Could you check a few things on this model? Use its own coordinates, in mm. A direction names the side the tool comes from. Give positions to 0.01 mm unless a question says otherwise; leave off trailing zeros. Order: outer loops, then holes, each group sorted by start corner. A loop starts at its lowest first (then second) coordinate and runs counter-clockwise, first axis right, second up. Notation, with made-up numbers: M 69,71 L 90,71 A14 cw 90,95 Z; hole C 7.5,7 d4. An arc over 180 degrees is marked long. Answer in a Markdown table with one row per item. Add a question column.
```python
from build123d import *

# Parameters (mm, degrees)
F1_DEPTH       = 101.6
F3_D           = 4.7752
F3_CBORE_D     = 9.525
F3_CBORE_DEPTH = 3.175
F5_D           = 4.7752
F5_CBORE_D     = 9.525
F5_CBORE_DEPTH = 3.175
F7_D           = 6.35
F8_SIZE        = 44.45
F9_R           = 12.7


with BuildPart() as f1:
    # F0 (on Front) → F1 (new body)
    with BuildSketch(Plane.XZ):
        Polygon((0, 9.525), (0, 0), (119.0752, 0), (119.0752, 10.549193), (68.2752, 10.549193), (68.2752, 55.613711), (61.9252, 55.613711), (61.9252, 10.139516), (57.15, 10.139516), (57.15, 55.40887), (50.8, 55.40887), (50.8, 9.525), align=None)
    extrude(amount=F1_DEPTH)

    # F3 (through all)
    with Locations(Plane.XY.offset(9.525)):
        with Locations((22.530584, -12.7), (24.763316, -88.9)):
            CounterBoreHole(F3_D / 2, F3_CBORE_D / 2, F3_CBORE_DEPTH)

    # F5 (through all)
    with Locations(Plane.XY.offset(10.549193)):
        with Locations((90.809768, -12.7), (93.242841, -88.9)):
            CounterBoreHole(F5_D / 2, F5_CBORE_D / 2, F5_CBORE_DEPTH)

    # F7 (through all)
    with Locations(Plane(origin=(50.8, 0, 0), x_dir=(0, -1, 0), z_dir=(-1, 0, 0))):
        with Locations((47.544591, 46.355)):
            Hole(F7_D / 2)

    # F8
    f8_edges = [f1.edges().sort_by_distance(p)[0] for p in [
        (53.975, 0, 55.40887),
        (53.975, -101.6, 55.40887),
        (65.1002, -101.6, 55.613711),
        (65.1002, 0, 55.613711),
    ]]
    chamfer(f8_edges, length=F8_SIZE)

    # F9
    f9_edges = [f1.edges().sort_by_distance(p)[0] for p in [
        (0, 0, 4.7625),
        (0, -101.6, 4.7625),
        (119.0752, -101.6, 5.274597),
        (119.0752, 0, 5.274597),
    ]]
    fillet(f9_edges, radius=F9_R)


solid = f1.part
```
1. Thinking about a two-plate mould opening in Y: for faces 1 (the flat face through (59, 0, 6)), 2 (the flat face through (59, -101.6, 6)), 3 (the flat face through (60, -50, 10.14)), 4 (the flat face through (95, -91, 7.374)), which applies, pulls with the +Y half, pulls with the -Y half, needs draft (parallel to the pull), parting line crosses it, or undercut?
2. Suppose I cut it at B-B on y = -68.5. List the corners of the cut face in (x, z) for me (3 decimals), plus the area to 3 significant figures.
3. Suppose I cut it at C-C on x = 48. List the corners of the cut face in (y, z) for me (3 decimals), plus the area to 3 significant figures.
4. Will these pins go through, and if not, where does the flat tip stop? P1, Ø1.5, axis at x = 51, z = 28, coming from the +Y side; P2, Ø7.5, axis at x = 23, y = -14, coming from the +Z side (3 decimals); P3, Ø5.5, axis at x = 22.53, y = -12.7, coming from the +Z side.
5. If I drill on line 1 along X through (y, z) = (-65.5, 38.5); line 2 along Y through (x, z) = (24, 4), over which ranges is the centre line in solid material (lowest first)? Write a range as [from, to].
6. Suppose I cut it at D-D on z = 14. List the corners of the cut face in (x, y) for me.
7. Suppose I cut it at A-A on z = 30. List the corners of the cut face in (x, y) for me.
8. For faces 5 (the flat face through (61.925, -50, 28)), 6 (the cylindrical face through (115.256, -3.622, 5.348)), 7 (the flat face through (26, -50, 9.525)), 8 (the flat face through (93, -15, 7.374)), 9 (the flat face through (68.275, -50, 28)), which set-ups out of +Z, -Z, +X, -X, +Y, -Y let a thin tool reach every point of the face, with its end or its side?
Findings below:
| question | item | result |
|---|---|---|
| 1 | face 1 | pulls with the +Y half |
| 1 | face 2 | pulls with the -Y half |
| 1 | face 3 | needs draft |
| 1 | face 4 | undercut |
| 2 | outline | M 0,0 L 119.075,0 L 119.075,10.549 L 68.275,10.549 L 68.275,44.264 L 61.925,44.264 L 61.925,10.14 L 57.15,10.14 L 57.15,44.059 L 50.8,44.059 L 50.8,9.525 L 0,9.525 Z |
| 2 | area | 1,630 mm2 |
| 3 | outline | M -101.6,0 L 0,0 L 0,9.525 L -101.6,9.525 Z |
| 3 | area | 968 mm2 |
| 4 | P1 | y = -16.29 |
| 4 | P2 | z = 9.525 |
| 4 | P3 | z = 6.35 |
| 5 | line 1 | [50.8, 57.15], [61.93, 68.28] |
| 5 | line 2 | [-101.6, -91.16], [-86.64, -14.58], [-10.82, 0] |
| 6 | outline | M 50.8,-98.56 L 57.15,-98.56 L 57.15,-3.04 L 50.8,-3.04 Z; M 61.93,-98.76 L 68.28,-98.76 L 68.28,-2.84 L 61.93,-2.84 Z |
| 7 | outline | M 50.8,-82.56 L 57.15,-82.56 L 57.15,-19.04 L 50.8,-19.04 Z; M 61.93,-82.76 L 68.28,-82.76 L 68.28,-18.84 L 61.93,-18.84 Z |
| 8 | face 5 | +Z, +Y, -Y |
| 8 | face 6 | +Z, -Z, +X, +Y |
| 8 | face 7 | +Z, -X, +Y, -Y |
| 8 | face 8 | +Z |
| 8 | face 9 | +Z, +X, +Y, -Y |
